```python
from build123d import *

# Parameters (mm, degrees)
F0_W     = 120
F0_H     = 70
F1_DEPTH = 100
F2_T     = -2.5
F4_DEPTH = 5
F5_R     = 2.5


with BuildPart() as f1:
    # F0 (on Front) → F1 (new body, symmetric)
    with BuildSketch(Plane.XZ):
        Rectangle(F0_W, F0_H)
    extrude(amount=F1_DEPTH, both=True)

    # F2
    f2_openings = [f1.faces().sort_by_distance(p)[0] for p in [
        (0, 0, 35),
    ]]
    offset(amount=F2_T, openings=f2_openings)

    # F3 (on Right) → F4 (join, symmetric)
    with BuildSketch(Plane.YZ):
        with BuildLine():
            Line((0, 35), (101, 35))
            Line((101, 35), (101, 0))
            Line((101, 0), (106, 0))
            Line((106, 0), (106, 50))
            ThreePointArc((106, 50), (101.259154, 60.976431), (90, 65))
            Line((90, 65), (65, 65))
            ThreePointArc((65, 65), (55.814413, 68.141459), (50.476312, 76.25))
            ThreePointArc((50.476312, 76.25), (48.696945, 78.952847), (45.635083, 80))
            Line((45.635083, 80), (0, 80))
            Line((0, 80), (-45.635083, 80))
            ThreePointArc((-45.635083, 80), (-48.696945, 78.952847), (-50.476312, 76.25))
            ThreePointArc((-50.476312, 76.25), (-55.814413, 68.141459), (-65, 65))
            Line((-65, 65), (-90, 65))
            ThreePointArc((-90, 65), (-101.259154, 60.976431), (-106, 50))
            Line((-106, 50), (-106, 0))
            Line((-106, 0), (-101, 0))
            Line((-101, 0), (-101, 35))
            Line((-101, 35), (-100, 35))
            Line((-100, 35), (0, 35))
        make_face()
        with BuildLine():
            Line((40, 47.5), (0, 47.5))
            Line((0, 47.5), (-40, 47.5))
            ThreePointArc((-40, 47.5), (-47.5, 55), (-40, 62.5))
            Line((-40, 62.5), (0, 62.5))
            Line((0, 62.5), (40, 62.5))
            ThreePointArc((40, 62.5), (47.5, 55), (40, 47.5))
        make_face(mode=Mode.SUBTRACT)
    extrude(amount=F4_DEPTH, both=True)

    # F5
    f5_edges = [f1.edges().sort_by_distance(p)[0] for p in [
        (5, 0, 47.5),
        (-5, 0, 47.5),
    ]]
    fillet(f5_edges, radius=F5_R)


solid = f1.part
```
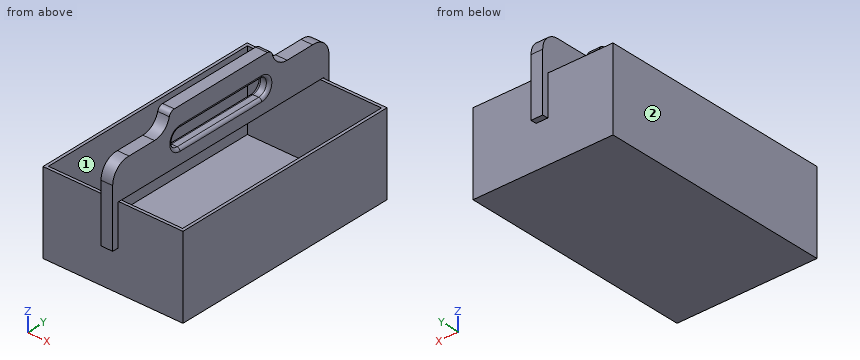
Input: part model. Units: mm. Frame: model coordinates. Face numbers are marked on the shaded views. A direction names the side the tool comes from. Coordinates: 2 decimals unless noted, no trailing zeros. Loops run counter-clockwise (first coordinate to the right, second up) from the corner with the lowest first, then second, coordinate; pieces in that order, holes last.
Q1. Section D-D, the plane y = -18. Give the number of separate pieces and of enclosed holes in the cut face, and give its area (3 significant figures).
Results are:
separate pieces: 3
enclosed holes: 0
area: 932 mm2
Q2. Contact query for flat-ended pins moving along their axis: pin 1 (1.5 mm diameter, centred on x = 39.5, z = -20, fed in from -Y); pin 2 (10 mm diameter, centred on x = 8.5, z = 55, fed in from -Y); pin 3 (16.5 mm diameter, centred on x = -36.5, y = 7, fed in from +Z). Output: stop coordinate, or through.
Results are:
pin 1: stops at y = -100
pin 2: stops at y = -105.93
pin 3: stops at z = -32.5
Q3. Set-up query: the marked faces 1 and 2. Return all of +Z, -Z, +X, -X, +Y, -Y with unobstructed straight access to the full face (end or side cutting, diameter ignored); none if empty.
Results are:
face 1: +Z
face 2: +Z, -Z, -X, +Y, -Y
Q4. Section B-B, the plane z = -26.5. Return the cut outline in (x, y).
Results are:
outline: (-60, -100) - (60, -100) - (60, 100) - (-60, 100) - close; hole (-57.5, -97.5) - (57.5, -97.5) - (57.5, 97.5) - (-57.5, 97.5) - close
Q5. Line query: line 1 along Y through (x, z) = (54.5, -13); line 2 along X through (y, z) = (-59, 23); line 3 along Z through (x, y) = (-5.5, 83). Output: solid intervals per line, ascending.
Results are:
line 1: y = -100 to -97.5, 97.5 to 100
line 2: x = -60 to -57.5, 57.5 to 60
line 3: z = -35 to -32.5
Q6. Section C-C, the plane x = -10. Return the cut outline in (y, z).
Results are:
outline: (-100, -35) - (100, -35) - (100, 35) - (97.5, 35) - (97.5, -32.5) - (-97.5, -32.5) - (-97.5, 35) - (-100, 35) - close
Q7. Section A-A, the plane z = 6. Return the cut outline in (x, y), and give its area (4 significant figures).
Results are:
outline: (-60, -100) - (60, -100) - (60, 100) - (-60, 100) - close; (-5, -106) - (5, -106) - (5, -101) - (-5, -101) - close; (-5, 101) - (5, 101) - (5, 106) - (-5, 106) - close; hole (-57.5, -97.5) - (57.5, -97.5) - (57.5, 97.5) - (-57.5, 97.5) - close
area: 1,675 mm2
